The model under review builds one solid part; all positions refer to its coordinate system, in mm. Face numbers are marked on the shaded views. A direction names the side the tool comes from. Coordinates: 2 decimals unless noted, no trailing zeros. Loops run counter-clockwise (first coordinate to the right, second up) from the corner with the lowest first, then second, coordinate; pieces in that order, holes last. Notation, with made-up numbers: (12.25, -19) - (36.25, -19) arc R14 cw to (36.25, -11) - close; hole circle Ø4 at (84, -26). An arc over 180 degrees is marked (long way). Use a Markdown table: item, result. Add a question column.
1) Add section A-A, the plane x = 273. Give the boundary of the cut face in (y, z) (3 decimals).
2) Add section C-C, the plane z = -110. Give the boundary of the cut face in (x, y), and give its area (3 significant figures).
3) Clearance check with flat-ended pins moving along their axes: pin 1 (11.5 mm diameter, centred on x = 649, y = -311, fed in from +Z); pin 2 (4 mm diameter, centred on y = -223.5, z = -81, fed in from -X); pin 3 (3 mm diameter, centred on y = -115.5, z = 44, fed in from -X). State where each tip first meets the part, or that it passes through.
4) Add section D-D, the plane x = 65. Give the boundary of the cut face in (y, z), and give its area (3 significant figures).
5) To check wall thickness, follow L1, parallel to Y at x = 152, z = 86.5; L2, parallel to Z at x = 286, y = -172 (3 decimals); L3, parallel to Y at x = 676.5, z = -121. State the ranges of each line that lie inside material, in increasing order. Write a range as [from, to].
6) Add section B-B, the plane y = -144. Give the boundary of the cut face in (x, z) (3 decimals), and give its area (3 significant figures).
7) The part is to be moulded in two halves that separate along Z. For the marked faces 1, 2, 3 and 4, say which applies: pulls with the +Z half, pulls with the -Z half, needs draft (parallel to the pull), parting line crosses it, or undercut.
8) For the marked faces 5, 6, 7 and 8, list the 3-axis set-ups (+Z, -Z, +X, -X, +Y, -Y) from which the entire face can be reached by the end or side of a thin tool; tool diameter is ignored.
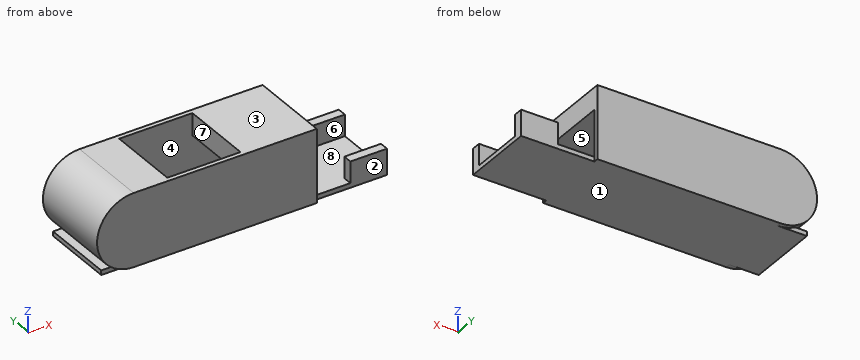
```python
from build123d import *

# Parameters (mm, degrees)
F1_DEPTH = 19.05
F2_W     = 304.8
F2_H     = 92.075
F3_DEPTH = 304.8
F4_W     = 304.8
F4_H     = 92.075
F5_DEPTH = 19.05
F6_W     = 304.8
F6_H     = 19.05
F7_DEPTH = 304.8
F8_W     = 152.4
F8_H     = 38.1
F9_DEPTH = 88.9


# Not quite as in the source:
# - a feature names something its author has since deleted; it is built from what else it names


with BuildPart() as f1:
    # F0 (on Front) → F1 (new body)
    with BuildSketch(Plane.XZ):
        with BuildLine():
            Line((457.2, -152.4), (457.2, 152.4))
            Line((457.2, 152.4), (-304.8, 152.4))
            ThreePointArc((-304.8, 152.4), (-197.0369265472, 107.7630734528), (-152.4, 0))
            ThreePointArc((-152.4, 0), (-197.0369262947, -107.7630732004), (-304.799999286, -152.4))
            Line((-304.799999286, -152.4), (457.2, -152.4))
        make_face()
        with BuildLine():
            ThreePointArc((-152.4, 0), (-197.0369265472, 107.7630734528), (-304.8, 152.4))
            ThreePointArc((-304.8, 152.4), (-412.5630734984, 107.7630734073), (-457.2, -1.288e-07))
            ThreePointArc((-457.2, -1.288e-07), (-412.5630731549, -107.7630737508), (-304.799999286, -152.4))
            ThreePointArc((-304.799999286, -152.4), (-197.0369262947, -107.7630732004), (-152.4, 0))
        make_face()
    extrude(amount=F1_DEPTH)

    # F2 (on face) → F3 (join)
    with BuildSketch(Plane.XZ.offset(19.05)):
        with Locations((304.8, 106.3625)):
            Rectangle(F2_W, F2_H)
    extrude(amount=F3_DEPTH)

    # F4 (on face) → F5 (join)
    with BuildSketch(Plane.XZ.offset(323.85)):
        with BuildLine():
            Line((152.4, 60.325), (152.4, 152.4))
            Line((152.4, 152.4), (-304.8, 152.4))
            ThreePointArc((-304.8, 152.4), (-197.0369265472, 107.7630734528), (-152.4, 0))
            ThreePointArc((-152.4, 0), (-197.0369262947, -107.7630732004), (-304.799999286, -152.4))
            Line((-304.799999286, -152.4), (457.2, -152.4))
            Line((457.2, -152.4), (457.2, 60.325))
            Line((457.2, 60.325), (152.4, 60.325))
        make_face()
        with Locations((304.8, 106.3625)):
            Rectangle(F4_W, F4_H)
        with BuildLine():
            ThreePointArc((-152.4, 0), (-197.0369265472, 107.7630734528), (-304.8, 152.4))
            ThreePointArc((-304.8, 152.4), (-412.5630734984, 107.7630734073), (-457.2, -1.288e-07))
            ThreePointArc((-457.2, -1.288e-07), (-412.5630731549, -107.7630737508), (-304.799999286, -152.4))
            ThreePointArc((-304.799999286, -152.4), (-197.0369262947, -107.7630732004), (-152.4, 0))
        make_face()
    extrude(amount=F5_DEPTH)

    # F6 (on face) → F7 (join, through all)
    with BuildSketch(Plane.XZ.offset(19.05)):
        with BuildLine():
            ThreePointArc((-304.799999286, -152.4), (-342.8999996543, -147.5606655798), (-378.5803327453, -133.35))
            Line((-378.5803327453, -133.35), (-427.4579864061, -133.35))
            Line((-427.4579864061, -133.35), (-427.4579864061, -152.4))
            Line((-427.4579864061, -152.4), (-304.799999286, -152.4))
        make_face()
        with BuildLine():
            Line((-152.4, 133.35), (-152.4, 152.4))
            Line((-152.4, 152.4), (-304.8, 152.4))
            ThreePointArc((-304.8, 152.4), (-266.7, 147.5606654905), (-231.0196672547, 133.35))
            Line((-231.0196672547, 133.35), (-152.4, 133.35))
        make_face()
        with BuildLine():
            ThreePointArc((-231.0196672547, 133.35), (-266.7, 147.5606654905), (-304.8, 152.4))
            Line((-304.8, 152.4), (-304.8, 133.35))
            Line((-304.8, 133.35), (-231.0196672547, 133.35))
        make_face()
        with BuildLine():
            Line((-304.8, 133.35), (-304.8, 152.4))
            ThreePointArc((-304.8, 152.4), (-452.3606654905, 38.1), (-378.5803327453, -133.35))
            Line((-378.5803327453, -133.35), (-304.7999985066, -133.35))
            ThreePointArc((-304.7999985066, -133.35), (-438.15, -7.467e-07), (-304.8, 133.35))
        make_face()
        with BuildLine():
            Line((-304.7999985066, -133.35), (-378.5803327453, -133.35))
            ThreePointArc((-378.5803327453, -133.35), (-342.8999996543, -147.5606655798), (-304.799999286, -152.4))
            ThreePointArc((-304.799999286, -152.4), (-266.6999996543, -147.5606654012), (-231.0196672547, -133.35))
            Line((-231.0196672547, -133.35), (-304.7999985066, -133.35))
        make_face()
        with Locations((609.6, -142.875)):
            Rectangle(F6_W, F6_H)
        with BuildLine():
            ThreePointArc((-231.0196672547, -133.35), (-266.6999996543, -147.5606654012), (-304.799999286, -152.4))
            Line((-304.799999286, -152.4), (457.2, -152.4))
            Line((457.2, -152.4), (457.2, -133.35))
            Line((457.2, -133.35), (-231.0196672547, -133.35))
        make_face()
    extrude(amount=F7_DEPTH)

    # F8 (on face) → F9 (join)
    with BuildSketch(Plane.XY.offset(-133.35)):
        with Locations((685.8, -38.1)):
            Rectangle(F8_W, F8_H)
        with Locations((685.8, -304.8)):
            Rectangle(F8_W, F8_H)
    extrude(amount=F9_DEPTH)


solid = f1.part
```
From the geometry:
| question | item | result |
|---|---|---|
| 1 | outline | (-342.9, -152.4) - (0, -152.4) - (0, 152.4) - (-342.9, 152.4) - close; hole (-323.85, -133.35) - (-19.05, -133.35) - (-19.05, 60.325) - (-323.85, 60.325) - close |
| 2 | outline | (-410.28, -342.9) - (457.2, -342.9) - (457.2, -323.85) - (-380.18, -323.85) - (-380.18, -19.05) - (457.2, -19.05) - (457.2, 0) - (-410.28, 0) - close; (609.6, -323.85) - (762, -323.85) - (762, -285.75) - (609.6, -285.75) - close; (609.6, -57.15) - (762, -57.15) - (762, -19.05) - (609.6, -19.05) - close |
| 2 | area | 53,800 mm^2 |
| 3 | pin 1 | stops at z = -44.45 |
| 3 | pin 2 | stops at x = -435.13 |
| 3 | pin 3 | stops at x = -451.15 |
| 4 | outline | (-342.9, -152.4) - (0, -152.4) - (0, 152.4) - (-19.05, 152.4) - (-19.05, -133.35) - (-323.85, -133.35) - (-323.85, 152.4) - (-342.9, 152.4) - close |
| 4 | area | 17,400 mm^2 |
| 5 | L1 | y = [-342.9, -323.85], [-19.05, 0] |
| 5 | L2 | z = [-152.4, -133.35], [60.325, 152.4] |
| 5 | L3 | y = [-323.85, -285.75], [-57.15, -19.05] |
| 6 | outline | (-427.458, -152.4) - (762, -152.4) - (762, -133.35) - (-304.8, -133.35) arc R133.35 cw to (-304.8, 133.35) - (-152.4, 133.35) - (-152.4, 152.4) - (-304.8, 152.4) arc R152.4 ccw to (-378.58, -133.35) - (-427.458, -133.35) - close; (152.4, 60.325) - (457.2, 60.325) - (457.2, 152.4) - (152.4, 152.4) - close |
| 6 | area | 61,200 mm^2 |
| 7 | face 1 | pulls with the -Z half |
| 7 | face 2 | needs draft |
| 7 | face 3 | pulls with the +Z half |
| 7 | face 4 | undercut |
| 8 | face 5 | +X |
| 8 | face 6 | +Z, +X |
| 8 | face 7 | +Z |
| 8 | face 8 | none |
